Read the model definition and answer for the solid it produces. Units are mm, in the model's axes. Face numbers are marked on the shaded views. A direction names the side the tool comes from. Round coordinates to 2 decimals unless told otherwise and drop trailing zeros. Order: outer loops, then holes, each group sorted by start corner. A loop starts at its lowest first (then second) coordinate and runs counter-clockwise, first axis right, second up.
from build123d import *


with BuildPart() as f1:
    # F0 (on Right) → F1 (revolve)
    with BuildSketch(Plane.YZ):
        with BuildLine():
            Line((1, 3), (1, 5))
            Line((1, 5), (0, 5))
            Line((0, 5), (0, 2.75))
            ThreePointArc((0, 2.75), (0.292893, 2.042893), (1, 1.75))
            Line((1, 1.75), (3.2, 1.75))
            ThreePointArc((3.2, 1.75), (3.907107, 2.042893), (4.2, 2.75))
            Line((4.2, 2.75), (4.2, 3.75))
            Line((4.2, 3.75), (3.2, 3.75))
            Line((3.2, 3.75), (3.2, 3))
            ThreePointArc((3.2, 3), (3.126777, 2.823223), (2.95, 2.75))
            Line((2.95, 2.75), (1.25, 2.75))
            ThreePointArc((1.25, 2.75), (1.073223, 2.823223), (1, 3))
        make_face()
    revolve(axis=Axis((0, 2.1, 0), (0, 1, 0)))


solid = f1.part
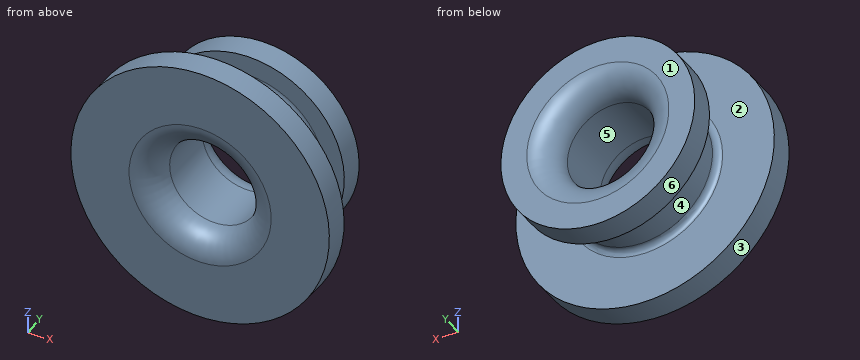
Q1. A cutting plane is placed at A-A, the plane x = 0. Give the vertices of the cut face in (y, z).
Outcome:
outline: (0, -5) - (1, -5) - (1, -3) arc R0.25 cw to (1.25, -2.75) - (2.95, -2.75) arc R0.25 cw to (3.2, -3) - (3.2, -3.75) - (4.2, -3.75) - (4.2, -2.75) arc R1 ccw to (3.2, -1.75) - (1, -1.75) arc R1 ccw to (0, -2.75) - close; (0, 2.75) arc R1 ccw to (1, 1.75) - (3.2, 1.75) arc R1 ccw to (4.2, 2.75) - (4.2, 3.75) - (3.2, 3.75) - (3.2, 3) arc R0.25 cw to (2.95, 2.75) - (1.25, 2.75) arc R0.25 cw to (1, 3) - (1, 5) - (0, 5) - close
Q2. For a pull along Y with two mould halves and no side action, classify the marked faces 1, 2 and 3 as released by +Y, released by -Y, zero draft, split by the parting line, or undercut.
Outcome:
face 1: released by +Y
face 2: undercut
face 3: zero draft
Q3. Flat-ended cylindrical pins translate along their axes: pin 1 (2 mm diameter, centred on y = 0.5, z = 2, fed in from -X); pin 2 (1 mm diameter, centred on x = 2.5, y = 2, fed in from -Z); pin 3 (2 mm diameter, centred on x = 0, z = -1.5, fed in from -Y). Find the tip coordinate at first contact, or state that the pin passes through.
Outcome:
pin 1: stops at x = -4.9
pin 2: stops at z = -1.89
pin 3: stops at y = 0.03
Q4. Straight lines are drawn through the part: probe 1 along X at (y, z) = (2.1, 0); probe 2 along Y at (x, z) = (1.5, -3); probe 3 along Y at (x, z) = (2.25, -4.25). For each, find the intervals that lie inside material, in ascending order.
Outcome:
probe 1: x = -2.75 to -1.75, 1.75 to 2.75
probe 2: y = 0 to 1, 3.2 to 4.2
probe 3: y = 0 to 1
Q5. A cutting plane is placed at C-C, the plane y = 3.8. Give the vertices of the cut face in (x, z), plus the area to 3 significant figures.
Outcome:
outline: circle Ø7.5 at (0, 0); hole circle Ø3.9 at (0, 0)
area: 32.2 mm2
Q6. A cutting plane is placed at D-D, the plane x = -3.5. Give the vertices of the cut face in (y, z).
Outcome:
outline: (0, -3.57) - (1, -3.57) - (1, 3.57) - (0, 3.57) - close; (3.2, -1.35) - (4.2, -1.35) - (4.2, 1.35) - (3.2, 1.35) - close
Q7. For the marked faces 4, 5 and 6, determine the directions among +Z, -Z, +X, -X, +Y, -Y from which every point of the face is accessible in a straight line to the end or side of a thin tool.
Outcome:
face 4: none
face 5: +Y, -Y
face 6: +Y
Q8. A cutting plane is placed at B-B, the plane z = 0. Give the vertices of the cut face in (x, y).
Outcome:
outline: (-5, 0) - (-2.75, 0) arc R1 ccw to (-1.75, 1) - (-1.75, 3.2) arc R1 ccw to (-2.75, 4.2) - (-3.75, 4.2) - (-3.75, 3.2) - (-3, 3.2) arc R0.25 cw to (-2.75, 2.95) - (-2.75, 1.25) arc R0.25 cw to (-3, 1) - (-5, 1) - close; (1.75, 1) arc R1 ccw to (2.75, 0) - (5, 0) - (5, 1) - (3, 1) arc R0.25 cw to (2.75, 1.25) - (2.75, 2.95) arc R0.25 cw to (3, 3.2) - (3.75, 3.2) - (3.75, 4.2) - (2.75, 4.2) arc R1 ccw to (1.75, 3.2) - close
